Autodesk Inventor part; units mm, degrees
ref_plane "YZ Plane" through (0, 0, 0) normal (1, 0, 0) x (0, 1, 0)
ref_plane "XZ Plane" through (0, 0, 0) normal (0, 1, 0) x (-1, 0, 0)
ref_plane "XY Plane" through (0, 0, 0) normal (0, 0, 1) x (1, 0, 0)
sketch "スケッチ1" plane through (0, 0, 0) normal (1, 0, 0) x (0, 1, 0)
  line L0 (10.2, 20) -> (10.2, 0)
  line L1 (10.2, 0) -> (9, 0)
  line L2 (9, 0) -> (9, -10)
  line L3 (9, -10) -> (14.8, -10)
  line L4 (0, -16) -> (0, 26)
  line L5 (10.2, 20) -> (14.8, 20)
  line L6 (14.8, 20) -> (14.8, -10)
  point P0 (0, 0)
  dimension "d2" = 10
  dimension "d3" = 10.2
  dimension "d12" = 9
  dimension "d14" = 14.8
  dimension "d15" = 20
revolve "回転1" add sketch "スケッチ1" angle 360 about axis through (0, 0, -10) along (0, 0, 1)
thread "ねじ1"
chamfer "面取り1" distance 23 distance2 3.6 1 edges at (0, -14.8, 20) measured on face at (1.1909, 14.752, 0)
chamfer "面取り2" distance 4 angle 45 1 edges at (0, -14.8, -10)
properties part number "rod330_end_cap" material "ステンレス鋼"
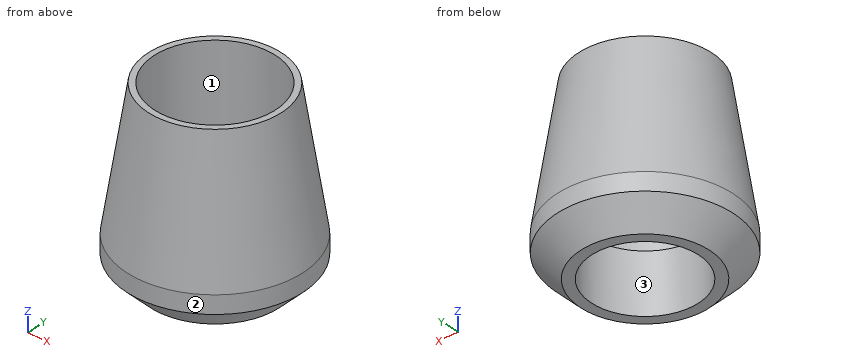
Build history of the part. All positions in model axes, mm. Face numbers are marked on the shaded views. Round coordinates to 2 decimals unless told otherwise and drop trailing zeros. Order: outer loops, then holes, each group sorted by start corner. A loop starts at its lowest first (then second) coordinate and runs counter-clockwise, first axis right, second up. Notation, with made-up numbers: (76.25, 71.5) -> (131.25, 71.5) arc R31 ccw to (131.25, 100.5) -> close; hole circle Ø10 at (13, 11). An arc over 180 degrees is marked (long way). Answer in a Markdown table with one row per item.
1) Band-saw the part on A-A on y = 0. Give the cut face in (x, z), and give its area (3 significant figures).
Values:
| item | result |
|---|---|
| outline | (-14.8, -6) -> (-10.8, -10) -> (-9, -10) -> (-9, 0) -> (-10.2, 0) -> (-10.2, 20) -> (-11.2, 20) -> (-14.8, -3) -> close; (9, -10) -> (10.8, -10) -> (14.8, -6) -> (14.8, -3) -> (11.2, 20) -> (10.2, 20) -> (10.2, 0) -> (9, 0) -> close |
| area | 201 mm2 |
2) Wall check: L1, parallel to Y at x = 0, z = -3.75; L2, parallel to Y at x = -5.25, z = -3.5. Give the ranges that are in metal, low to high.
Values:
| item | result |
|---|---|
| L1 | -14.8 to -9, 9 to 14.8 |
| L2 | -13.84 to -7.31, 7.31 to 13.84 |
3) Mould opens along X. For the marked faces 1, 2 and 3 say: released by +X, released by -X, zero draft, split by the parting line, or undercut.
Values:
| item | result |
|---|---|
| face 1 | undercut |
| face 2 | split by the parting line |
| face 3 | undercut |
4) Band-saw the part on D-D on z = 4.5. Give the cut face in (x, y).
Values:
| item | result |
|---|---|
| outline | circle Ø27.25 at (0, 0); hole circle Ø20.4 at (0, 0) |
5) Band-saw the part on C-C on z = -4.25. Give the cut face in (x, y), and give its area (3 significant figures).
Values:
| item | result |
|---|---|
| outline | circle Ø29.6 at (0, 0); hole circle Ø18 at (0, 0) |
| area | 434 mm2 |
6) Pin check, flat tips, straight feed: P1, Ø2, axis at x = -1, z = -1, coming from the +Y side; P2, Ø1.5, axis at x = -7.5, z = 7.5, coming from the +Y side; P3, Ø6, axis at y = 11.5, z = 13, coming from the -X side. Stop position of each tip, or through.
Values:
| item | result |
|---|---|
| P1 | y = 14.62 |
| P2 | y = 11.31 |
| P3 | x = -8.96 |
